```python
from build123d import *

# Parameters (mm, degrees)
F1_DEPTH = 33.02
F1_TAPER = -26.56505118
F3_DEPTH = 33.02
F3_TAPER = -26.56505118
F5_DEPTH = 50.8
F6_SIZE2 = 16.7177543947
F6_SIZE  = 9.652
F8_DEPTH = 50.8
F9_SIZE2 = 16.51
F9_SIZE  = 9.5320529443


with BuildPart() as f1:
    # F0 (on Top) → F1 (new body)
    with BuildSketch(Plane.XY):
        Polygon((12.0784177569, -3.9245158286), (7.4648727041, 10.2745158286), (-7.4648727041, 10.2745158286), (-12.0784177569, -3.9245158286), (0, -12.7), align=None)
    extrude(amount=F1_DEPTH, taper=F1_TAPER)

    # F2 (on face) → F3 (intersect)
    with BuildSketch(Plane.XY.offset(33.02)):
        Polygon((7.4648727041, -10.2745158286), (12.0784177569, 3.9245158286), (0, 12.7), (-12.0784177569, 3.9245158286), (-7.4648727041, -10.2745158286), align=None)
    extrude(amount=-F3_DEPTH, taper=F3_TAPER, mode=Mode.INTERSECT)

    # F4 (on face) → F5 (join)
    with BuildSketch(Plane.XY.offset(33.02)):
        Polygon((-12.0784177569, 3.9245158286), (-7.4648727041, -10.2745158286), (7.4648727041, -10.2745158286), (12.0784177569, 3.9245158286), (0, 12.7), align=None)
    extrude(amount=F5_DEPTH)

    # F6
    f6_edges = [f1.edges().sort_by_distance(p)[0] for p in [
        (9.771645, -3.175, 83.82),
        (0, -10.274516, 83.82),
        (-9.771645, -3.175, 83.82),
        (-6.039209, 8.312258, 83.82),
        (6.039209, 8.312258, 83.82),
    ]]
    f6_side = f1.faces().sort_by_distance((0, 0, 83.82))[0]
    chamfer(f6_edges, length=F6_SIZE, length2=F6_SIZE2, reference=f6_side)

    # F7 (on face) → F8 (join)
    with BuildSketch(Plane(origin=(0, 0, 0), x_dir=(1, 0, 0), z_dir=(0, 0, -1))):
        Polygon((0, 12.7), (-12.0784177569, 3.9245158286), (-7.4648727041, -10.2745158286), (7.4648727041, -10.2745158286), (12.0784177569, 3.9245158286), align=None)
    extrude(amount=F8_DEPTH)

    # F9
    f9_edges = [f1.edges().sort_by_distance(p)[0] for p in [
        (-9.771645, 3.175, -50.8),
        (0, 10.274516, -50.8),
        (9.771645, 3.175, -50.8),
        (6.039209, -8.312258, -50.8),
        (-6.039209, -8.312258, -50.8),
    ]]
    f9_side = f1.faces().sort_by_distance((0, 0, -50.8))[0]
    chamfer(f9_edges, length=F9_SIZE, length2=F9_SIZE2, reference=f9_side)


solid = f1.part
```
Part model, mm, in its own coordinate system. A direction names the side the tool comes from. Round coordinates to 2 decimals unless told otherwise and drop trailing zeros. Loops run counter-clockwise (first coordinate to the right, second up) from the corner with the lowest first, then second, coordinate; pieces in that order, holes last. Notation, with made-up numbers: (35.5, 21.25) -> (70.5, 21.25) arc R12 cw to (70.5, 28.25) -> close; hole circle Ø9 at (49.25, 83.25). An arc over 180 degrees is marked (long way). Use a Markdown table: item, result.
1) Cut at B-B, the plane z = -36.5. List the corners of the cut face in (x, y).
The answers:
| item | result |
|---|---|
| outline | (-10.58, -3.44) -> (0, -11.12) -> (10.58, -3.44) -> (6.54, 9) -> (-6.54, 9) -> close |
2) Cut at A-A, the plane z = 65.5. List the corners of the cut face in (x, y), and give its area (3 significant figures).
The answers:
| item | result |
|---|---|
| outline | (-12.08, 3.92) -> (-7.46, -10.27) -> (7.46, -10.27) -> (12.08, 3.92) -> (0, 12.7) -> close |
| area | 383 mm2 |
3) Tool access for faces 1 (the flat face through (-5.955, 8.374, 49.823)), 2 (the flat face through (0, 10.275, -17)), 3 (the flat face through (0, -10.275, 50)): list every direction of +Z, -Z, +X, -X, +Y, -Y with a clear straight run to the whole face (end or side of a thin tool).
The answers:
| item | result |
|---|---|
| face 1 | +Z, -X, +Y |
| face 2 | -Z, +X, -X, +Y |
| face 3 | +Z, +X, -X, -Y |
4) Probe line 1 (Y direction, x = 12.5, z = 14); line 2 (Y direction, x = 8, z = 15); line 3 (Z direction, x = 0.5, y = 13). List the from-to ranges inside material, lowest first. Write a range as [from, to].
The answers:
| item | result |
|---|---|
| line 1 | y = [-12.27, 15.37] |
| line 2 | y = [-16.16, 17.77] |
| line 3 | z = [5.45, 31.95] |
5) Drop flat-ended pins along their axis: pin 1 Ø4 at (x, z) = (-15.5, 6.5) entering from -Y; pin 2 Ø5 at (y, z) = (14, 33) entering from +X; pin 3 Ø16.5 at (x, z) = (-3.5, 50) entering from -Y. Give the stop position or say it passes through.
The answers:
| item | result |
|---|---|
| pin 1 | stops at y = -7.36 |
| pin 2 | stops at x = 2.27 |
| pin 3 | stops at y = -10.27 |
